Could you check a few things on this model? Use its own coordinates, in mm. A direction names the side the tool comes from. Round coordinates to 2 decimals unless told otherwise and drop trailing zeros. Write each loop counter-clockwise with the first axis right and the second up, starting at its lowest first coordinate (ties: lowest second). Pieces come first, ordered by that corner, then holes. Notation, with made-up numbers: (13, 21.5) - (27, 21.5) arc R9 ccw to (27, 35.5) - close; hole circle Ø11 at (76.25, 34). An arc over 180 degrees is marked (long way). Put each result on its own line as item: value.
from build123d import *

# Parameters (mm, degrees)
F0_W     = 63.5
F0_H     = 63.5
F0_W_2   = 57.5
F0_H_2   = 57.5
F1_DEPTH = 140
F2_R     = 10
F3_DEPTH = 3


# Not quite as in the source:
# - a feature names something its author has since deleted; it is built from what else it names


with BuildPart() as f1:
    # F0 (on Top) → F1 (new body)
    with BuildSketch(Plane.XY):
        with Locations((2.4368530139, 1.7202482249)):
            Rectangle(F0_W, F0_H)
        with Locations((2.4368530139, 1.7202482249)):
            Rectangle(F0_W_2, F0_H_2, mode=Mode.SUBTRACT)
    extrude(amount=F1_DEPTH)

    # F2 (on face) → F3 (cut)
    with BuildSketch(Plane(origin=(-29.3131469861, 0, 0), x_dir=(0, -1, 0), z_dir=(-1, 0, 0))):
        with Locations((-1.7202482249, 20)):
            Circle(F2_R)
    extrude(amount=-F3_DEPTH, mode=Mode.SUBTRACT)


solid = f1.part
(1) Imagine slicing it at B-B, the plane x = 18.5. List the corners of the cut face in (y, z) for me.
Values found:
outline: (-30.03, 0) - (-27.03, 0) - (-27.03, 140) - (-30.03, 140) - close; (30.47, 0) - (33.47, 0) - (33.47, 140) - (30.47, 140) - close
(2) Imagine slicing it at A-A, the plane y = 14. List the corners of the cut face in (x, z) for me.
Values found:
outline: (-29.31, 0) - (-26.31, 0) - (-26.31, 140) - (-29.31, 140) - close; (31.19, 0) - (34.19, 0) - (34.19, 140) - (31.19, 140) - close
(3) For faces 1 (the face through (-27.834, 3.022, 29.915)), 2 (the face through (31.187, 1, 69)), 3 (the face through (0, -29, 0)), which set-ups out of +Z, -Z, +X, -X, +Y, -Y let a thin tool reach every point of the face, with its end or its side?
Values found:
face 1: -X
face 2: +Z, -Z
face 3: -Z, +X, -X, +Y, -Y
(4) Imagine slicing it at C-C, the plane z = 50.5. List the corners of the cut face in (x, y) for me.
Values found:
outline: (-29.31, -30.03) - (34.19, -30.03) - (34.19, 33.47) - (-29.31, 33.47) - close; hole (-26.31, -27.03) - (31.19, -27.03) - (31.19, 30.47) - (-26.31, 30.47) - close
(5) Please list where these lines run through material, in increasing order: probe 1 along Y at (x, z) = (-14.5, 120.5); probe 2 along X at (y, z) = (27.5, 131). Write a range as from..to.
Values found:
probe 1: y = -30.03..-27.03, 30.47..33.47
probe 2: x = -29.31..-26.31, 31.19..34.19
(6) If we mould it in two halves opening along X, with no side actions, what happens to faces 4 (the face through (0, -29, 140)), 5 (the face through (34.187, 1, 69)), 6 (the face through (2, -27.03, 69))? For each: pulls with the +X half, pulls with the -X half, needs draft (parallel to the pull), parting line crosses it, or undercut.
Values found:
face 4: needs draft
face 5: pulls with the +X half
face 6: undercut
(7) Imagine slicing it at D-D, the plane z = 20. List the corners of the cut face in (x, y) for me.
Values found:
outline: (-29.31, -30.03) - (34.19, -30.03) - (34.19, 33.47) - (-29.31, 33.47) - (-29.31, 11.72) - (-26.31, 11.72) - (-26.31, 30.47) - (31.19, 30.47) - (31.19, -27.03) - (-26.31, -27.03) - (-26.31, -8.28) - (-29.31, -8.28) - close
